from build123d import *

# Parameters (mm, degrees)
SKETCH1_R           = 6.25
SKETCH1_R_2         = 3.75
BOSS_EXTRUDE2_DEPTH = 50
FILLET1_R           = 0.5
FILLET2_R           = 0.5


with BuildPart() as part:
    # Sketch1 → Boss-Extrude2 (new body)
    with BuildSketch(Plane(origin=(0, 0, 0), x_dir=(0, 0, -1), z_dir=(1, 0, 0))):
        Circle(SKETCH1_R)
        Circle(SKETCH1_R_2, mode=Mode.SUBTRACT)
    extrude(amount=BOSS_EXTRUDE2_DEPTH)

    # Fillet1
    fillet1_edges = [part.edges().sort_by_distance(p)[0] for p in [
        (0, 0, 6.25),
    ]]
    fillet(fillet1_edges, radius=FILLET1_R)

    # Fillet2
    fillet2_edges = [part.edges().sort_by_distance(p)[0] for p in [
        (50, 0, 6.25),
    ]]
    fillet(fillet2_edges, radius=FILLET2_R)


solid = part.part
Source: CAD feature listing. Evaluate the final solid. Frame: model axes, mm. Coordinates: 2 decimals unless noted, no trailing zeros. Loops run counter-clockwise (first coordinate to the right, second up) from the corner with the lowest first, then second, coordinate; pieces in that order, holes last. Notation, with made-up numbers: (-32, 68.5) - (-19, 68.5) arc R10 cw to (-19, 81.5) - close; hole circle Ø9 at (84.5, 11.25). An arc over 180 degrees is marked (long way). Return JSON: item names as keys, results as strings.
Q1. Material intervals for line 1 along Y through (x, z) = (39, 0); line 2 along Z through (x, y) = (38.5, 1); line 3 along Z through (x, y) = (8.5, -1.5), sorted ascending.
Results:
{"line 1": "-6.25 to -3.75, 3.75 to 6.25", "line 2": "-6.17 to -3.61, 3.61 to 6.17", "line 3": "-6.07 to -3.44, 3.44 to 6.07"}
Q2. Section C-C, the plane x = 43.5. Return loops of the section in (y, z).
Results:
{"outline": "circle Ø12.5 at (0, 0); hole circle Ø7.5 at (0, 0)"}
Q3. Mould query, pull axis Y, two halves, no side actions, for faces 1 (the flat face through (50, -4, 0)), 2 (the cylindrical face through (24.66, 1.88, -5.96)), 3 (the cylindrical face through (24.65, 0.165, 3.746)). Classes: released by +Y, released by -Y, zero draft, split by the parting line, or undercut.
Results:
{"face 1": "zero draft", "face 2": "split by the parting line", "face 3": "undercut"}
Q4. Section A-A, the plane z = 0. Return loops of the section in (x, y), plus the area to 3 significant figures.
Results:
{"outline": "(0, -5.75) arc R0.5 ccw to (0.5, -6.25) - (49.5, -6.25) arc R0.5 ccw to (50, -5.75) - (50, -3.75) - (0, -3.75) - close; (0, 3.75) - (50, 3.75) - (50, 5.75) arc R0.5 ccw to (49.5, 6.25) - (0.5, 6.25) arc R0.5 ccw to (0, 5.75) - close", "area": "250 mm2"}
Q5. Contact query for flat-ended pins moving along their axis: P1, Ø3, axis at x = 44, z = -2.5, coming from the -Y side; P2, Ø6, axis at x = 21.5, z = 4, coming from the +Y side; P3, Ø1, axis at y = 1, z = 2, coming from the +X side; P4, Ø4, axis at x = 21, y = -3, coming from the +Z side. Output: stop coordinate, or through.
Results:
{"P1": "y = -6.17", "P2": "y = 6.17", "P3": "through", "P4": "z = 6.17"}
